from build123d import *

# Parameters (mm, degrees)
SKETCH1_W           = 120
SKETCH1_H           = 30
BOSS_EXTRUDE1_DEPTH = 3
SKETCH3_R           = 1
CUT_EXTRUDE1_DEPTH  = 4
FILLET1_R           = 14


with BuildPart() as part:
    # Sketch1 → Boss-Extrude1 (new body)
    with BuildSketch(Plane(origin=(0, 0, 0), x_dir=(1, 0, 0), z_dir=(0, 1, 0))):
        with Locations((60, 15)):
            Rectangle(SKETCH1_W, SKETCH1_H)
    extrude(amount=BOSS_EXTRUDE1_DEPTH)

    # Sketch3 → Cut-Extrude1 (cut, through all)
    with BuildSketch(Plane(origin=(0, 3, 0), x_dir=(1, 0, 0), z_dir=(0, 1, 0))):
        with Locations((20, 15)):
            Circle(SKETCH3_R)
    extrude(amount=-CUT_EXTRUDE1_DEPTH, mode=Mode.SUBTRACT)

    # Fillet1
    fillet1_edges = [part.edges().sort_by_distance(p)[0] for p in [
        (0, 1.5, -30),
        (0, 1.5, 0),
    ]]
    fillet(fillet1_edges, radius=FILLET1_R)


solid = part.part
Geometry check sheet. Reference: the model listing, model coordinates, mm. Give positions to 0.01 mm unless a question says otherwise; leave off trailing zeros. Order: outer loops, then holes, each group sorted by start corner. A loop starts at its lowest first (then second) coordinate and runs counter-clockwise, first axis right, second up. Notation, with made-up numbers: M 2.5,44.5 L 38.5,44.5 A23 cw 38.5,63.5 Z; hole C -9.5,52 d7. An arc over 180 degrees is marked long. Use a Markdown table: item, result.
Item 1: Draft check along Z on faces 1 (the flat face through (66, 1, 0)), 2 (the flat face through (59, 0, -15)), 3 (the cylindrical face through (20, 2, -14)). Enter one of: +Z half, -Z half, draft (parallel to the pull), parting line (faces both ways), or undercut.
Answers follow:
| item | result |
|---|---|
| face 1 | +Z half |
| face 2 | draft |
| face 3 | undercut |
Item 2: Section check D-D (z = -6.75). Record the cut outline in (x, y), and give its area (3 significant figures).
Answers follow:
| item | result |
|---|---|
| outline | M 2.02,0 L 120,0 L 120,3 L 2.02,3 Z |
| area | 354 mm2 |
Item 3: Section check A-A (z = -15). Record the cut outline in (x, y), and give its area (3 significant figures).
Answers follow:
| item | result |
|---|---|
| outline | M 0,0 L 19,0 L 19,3 L 0,3 Z; M 21,0 L 120,0 L 120,3 L 21,3 Z |
| area | 354 mm2 |
Item 4: Section check C-C (x = 20). Record the cut outline in (y, z), and give its area (3 significant figures).
Answers follow:
| item | result |
|---|---|
| outline | M 0,-30 L 3,-30 L 3,-16 L 0,-16 Z; M 0,-14 L 3,-14 L 3,0 L 0,0 Z |
| area | 84.0 mm2 |
Item 5: Depth check by flat-ended pin: P1, Ø3, axis at x = 30, z = -11, coming from the -Y side; P2, Ø1.5, axis at y = 1.5, z = -17.5, coming from the -X side. Enter the tip coordinate at first touch or a pass-through.
Answers follow:
| item | result |
|---|---|
| P1 | stops at y = 0 |
| P2 | stops at x = 0.02 |
Item 6: Section check B-B (y = 1.3). Record the cut outline in (x, z), and give its area (3 significant figures).
Answers follow:
| item | result |
|---|---|
| outline | M 0,-16 A14 ccw 14,-30 L 120,-30 L 120,0 L 14,0 A14 ccw 0,-14 Z; hole C 20,-15 d2 |
| area | 3,510 mm2 |
Item 7: Material ranges on line 1 along Z through (x, y) = (20, 2.2); line 2 along X through (y, z) = (1.05, -15); line 3 along X through (y, z) = (0.65, -15.5), recorded low to high.
Answers follow:
| item | result |
|---|---|
| line 1 | z = -30 to -16, -14 to 0 |
| line 2 | x = 0 to 19, 21 to 120 |
| line 3 | x = 0 to 19.13, 20.87 to 120 |
